```python
from build123d import *

# Parameters (mm, degrees)
F0_R     = 1.9
F1_DEPTH = 0.9
F2_DEPTH = 4.5
F3_DEPTH = 3.3


with BuildPart() as f1:
    # F0 (on Top) → F1 (new body)
    with BuildSketch(Plane.XY):
        with BuildLine():
            Line((-0.3, 2.6000520814), (-3.8955825641, 2.5999907979))
            ThreePointArc((-3.8955825641, 2.5999907979), (-6.5018304859, -0.0590002136), (-3.7776200645, -2.5969992302))
            Line((-3.7776200645, -2.5969992302), (-0.3, -2.6039384091))
            Line((-0.3, -2.6039384091), (-0.3, 2.6000520814))
        make_face()
        with Locations((-3.9025, 0)):
            Circle(F0_R, mode=Mode.SUBTRACT)
        with BuildLine():
            ThreePointArc((-3.7776200645, -2.5969992302), (-6.5018304859, -0.0590002136), (-3.8955825641, 2.5999907979))
            Line((-3.8955825641, 2.5999907979), (-0.3, 2.6000520814))
            Line((-0.3, 2.6000520814), (-0.3, 3.2423396327))
            Line((-0.3, 3.2423396327), (-3.8955825641, 3.2499926383))
            ThreePointArc((-3.8955825641, 3.2499926383), (-7.1524938186, 0.0063386972), (-3.9082599583, -3.2499948958))
            Line((-3.9082599583, -3.2499948958), (-0.3, -3.2563898065))
            Line((-0.3, -3.2563898065), (-0.3, -2.6039384091))
            Line((-0.3, -2.6039384091), (-3.7776200645, -2.5969992302))
        make_face()
        with Locations((-3.9025, 0)):
            Circle(F0_R)
    extrude(amount=F1_DEPTH)

    # F0 (on Top) → F2 (join)
    with BuildSketch(Plane.XY):
        with BuildLine():
            Line((-0.3, 2.6000520814), (-3.8955825641, 2.5999907979))
            ThreePointArc((-3.8955825641, 2.5999907979), (-6.5018304859, -0.0590002136), (-3.7776200645, -2.5969992302))
            Line((-3.7776200645, -2.5969992302), (-0.3, -2.6039384091))
            Line((-0.3, -2.6039384091), (-0.3, 2.6000520814))
        make_face()
        with Locations((-3.9025, 0)):
            Circle(F0_R, mode=Mode.SUBTRACT)
        with Locations((-3.9025, 0)):
            Circle(F0_R)
    extrude(amount=F2_DEPTH)


with BuildPart() as f1b:
    # F0 (on Top) → F1, piece 2 (new body)
    with BuildSketch(Plane.XY):
        with BuildLine():
            Line((0.3, 2.5976768642), (0.3, -2.6051356381))
            Line((0.3, -2.6051356381), (4.0469650256, -2.612612263))
            ThreePointArc((4.0469650256, -2.612612263), (6.5020444574, 0.0503066263), (3.913198154, 2.5833733141))
            Line((3.913198154, 2.5833733141), (0.3, 2.5976768642))
        make_face()
        with Locations((3.9029056272, -0.0166063135)):
            Circle(F0_R, mode=Mode.SUBTRACT)
        with BuildLine():
            Line((0.3, -2.6051356381), (0.3, -3.257453185))
            Line((0.3, -3.257453185), (4.0313724183, -3.2640662876))
            ThreePointArc((4.0313724183, -3.2640662876), (7.1522718987, 0.0475718266), (3.9030412728, 3.2333936837))
            Line((3.9030412728, 3.2333936837), (0.3, 3.2410625647))
            Line((0.3, 3.2410625647), (0.3, 2.5976768642))
            Line((0.3, 2.5976768642), (3.913198154, 2.5833733141))
            ThreePointArc((3.913198154, 2.5833733141), (6.5020444574, 0.0503066263), (4.0469650256, -2.612612263))
            Line((4.0469650256, -2.612612263), (0.3, -2.6051356381))
        make_face()
        with Locations((3.9029056272, -0.0166063135)):
            Circle(F0_R)
    extrude(amount=F1_DEPTH)

    # F0 (on Top) → F2, piece 2 (join)
    with BuildSketch(Plane.XY):
        with BuildLine():
            Line((0.3, 2.5976768642), (0.3, -2.6051356381))
            Line((0.3, -2.6051356381), (4.0469650256, -2.612612263))
            ThreePointArc((4.0469650256, -2.612612263), (6.5020444574, 0.0503066263), (3.913198154, 2.5833733141))
            Line((3.913198154, 2.5833733141), (0.3, 2.5976768642))
        make_face()
        with Locations((3.9029056272, -0.0166063135)):
            Circle(F0_R, mode=Mode.SUBTRACT)
        with Locations((3.9029056272, -0.0166063135)):
            Circle(F0_R)
    extrude(amount=F2_DEPTH)


with BuildPart() as f3_tool:
    # F0 (on Top) → F3 (new body)
    with BuildSketch(Plane.XY):
        with Locations((-3.9025, 0)):
            Circle(F0_R)
        with Locations((3.9029056272, -0.0166063135)):
            Circle(F0_R)
    extrude(amount=F3_DEPTH)


with BuildPart() as f1_1:
    add(f1.part)

    # F3: cut by f3_tool
    add(f3_tool.part, mode=Mode.SUBTRACT)


with BuildPart() as f1b_1:
    add(f1b.part)

    # F3: cut by f3_tool
    add(f3_tool.part, mode=Mode.SUBTRACT)


solid = f1b_1.part
```
Input: part model. Units: mm. Frame: model coordinates. A direction names the side the tool comes from. Coordinates: 2 decimals unless noted, no trailing zeros. Order: outer loops, then holes, each group sorted by start corner. A loop starts at its lowest first (then second) coordinate and runs counter-clockwise, first axis right, second up. Notation, with made-up numbers: (-27, 57) - (-22, 57) arc R20 cw to (-22, 84) - close; hole circle Ø11 at (-3, 25.25). An arc over 180 degrees is marked (long way). Return JSON: item names as keys, results as strings.
Q1. Access query for faces 1 (the flat face through (2, 1, 0)), 2 (the cylindrical face through (2.005, 0.067, 1.627)), 3 (the cylindrical face through (6.503, -0.006, 2.675)). Directions: +Z, -Z, +X, -X, +Y, -Y. A direction counts if a zero-diameter tool reaches every point of the face in a straight line with its end or side. Return the directions, or none.
The answers:
{"face 1": "-Z, +X, -X, +Y, -Y", "face 2": "-Z", "face 3": "+Z, +X"}
Q2. Cut plane B-B (x = 4.5). Return loops of the section in (y, z), then the cut area to 3 significant figures.
The answers:
{"outline": "(-3.21, 0) - (-1.82, 0) - (-1.82, 3.3) - (1.79, 3.3) - (1.79, 0) - (3.18, 0) - (3.18, 0.9) - (2.51, 0.9) - (2.51, 4.5) - (-2.55, 4.5) - (-2.55, 0.9) - (-3.21, 0.9) - close", "area": "12.1 mm2"}
Q3. First-contact query: pin 1 (1.5 mm diameter, centred on x = 5.5, z = 3, fed in from +Y); pin 2 (1.1 mm diameter, centred on x = 4.5, y = 0.5, fed in from -Z); pin 3 (1.5 mm diameter, centred on y = -2, z = 3, fed in from +X). Flat tips, straight axial feed; report the tip coordinate or a pass-through.
The answers:
{"pin 1": "stops at y = 2.44", "pin 2": "stops at z = 3.3", "pin 3": "stops at x = 6.19"}
Q4. Cut plane A-A (y = -1). Return loops of the section in (x, z).
The answers:
{"outline": "(0.3, 0) - (2.28, 0) - (2.28, 3.3) - (5.53, 3.3) - (5.53, 0) - (7, 0) - (7, 0.9) - (6.31, 0.9) - (6.31, 4.5) - (0.3, 4.5) - close"}
Q5. Cut plane C-C (z = 2.45). Return loops of the section in (x, y).
The answers:
{"outline": "(0.3, -2.61) - (4.05, -2.61) arc R2.6 ccw to (3.91, 2.58) - (0.3, 2.6) - close; hole circle Ø3.8 at (3.9, -0.02)"}
Q6. Draft query along Z for faces 4 (the cylindrical face through (7.153, -0.023, 0.444)), 5 (the flat face through (6, -2, 0.9)), 6 (the flat face through (4, 0, 3.3)). Return one class per face: +Z half, -Z half, draft (parallel to the pull), parting line (faces both ways), or undercut.
The answers:
{"face 4": "draft", "face 5": "+Z half", "face 6": "-Z half"}
Q7. Ray query, probe 1 along Z at (x, y) = (5, -0.5); probe 2 along Y at (x, z) = (3.75, 3.4); probe 3 along X at (y, z) = (0.5, 2.7). Return the intervals inside material, ascending.
The answers:
{"probe 1": "z = 3.3 to 4.5", "probe 2": "y = -2.61 to 2.58", "probe 3": "x = 0.3 to 2.07, 5.73 to 6.45"}
